For this review, use the dimensioned drawing (mm, ordinates from the lowest corner) and the shaded views. A direction names the side the tool comes from. Give positions to 0.01 mm unless a question says otherwise; leave off trailing zeros. Loops run counter-clockwise (first coordinate to the right, second up) from the corner with the lowest first, then second, coordinate; pieces in that order, holes last. Notation, with made-up numbers: M 76,59 L 119,59 A25 cw 119,86 Z; hole C 73.25,73.5 d6. An arc over 180 degrees is marked long. Return JSON: item names as keys, results as strings.
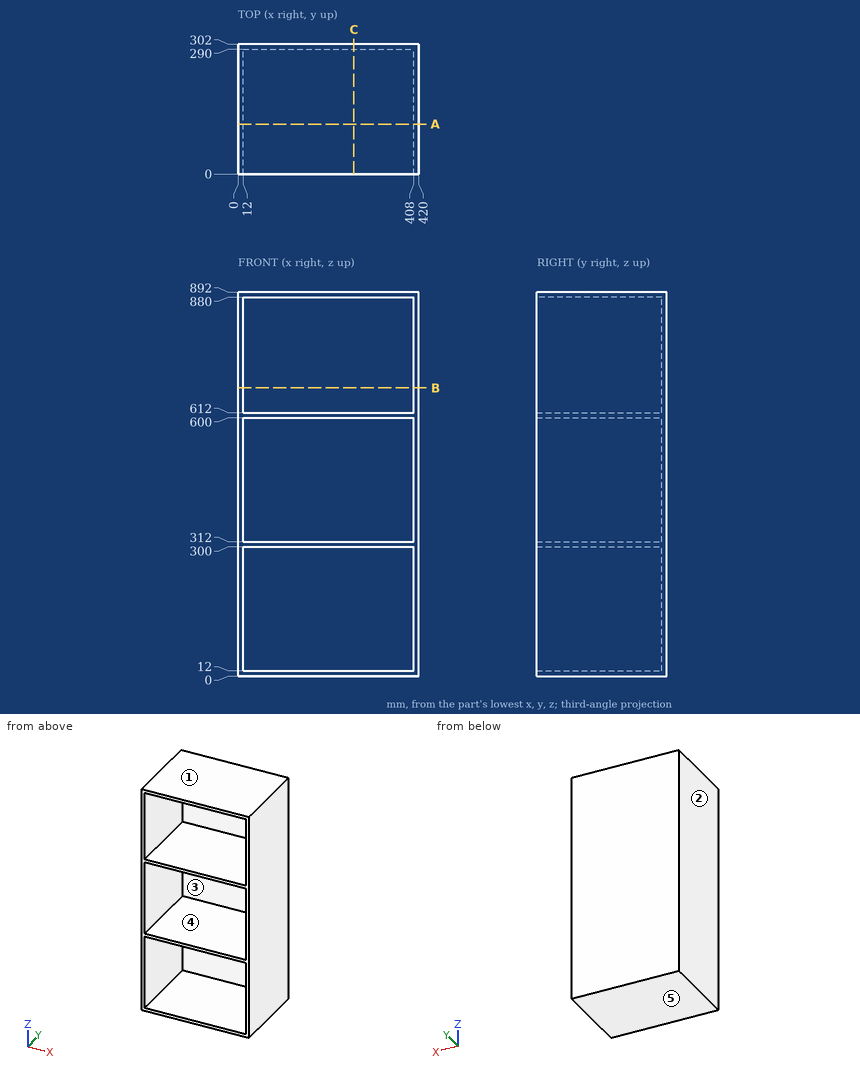
1) Consider section C-C on x = 269. Write out the cut boundary in (y, z).
From the geometry:
{"outline": "M 0,0 L 302,0 L 302,892 L 0,892 L 0,880 L 290,880 L 290,612 L 0,612 L 0,600 L 290,600 L 290,312 L 0,312 L 0,300 L 290,300 L 290,12 L 0,12 Z"}
2) Consider section B-B on z = 669.5. Write out the cut boundary in (x, y).
From the geometry:
{"outline": "M 0,0 L 12,0 L 12,290 L 408,290 L 408,0 L 420,0 L 420,302 L 0,302 Z"}
3) Tool access review of the marked faces 4 and 5: name each direction out of +Z, -Z, +X, -X, +Y, -Y from which nothing blocks a thin tool from reaching the whole face with its end or side.
From the geometry:
{"face 4": "-Y", "face 5": "-Z, +X, -X, +Y, -Y"}
4) Insertion check: pin 1 (1.5 mm diameter, centred on x = 259.5, y = 248, fed in from -Z); pin 2 (5 mm diameter, centred on x = 372.5, z = 712.5, fed in from -Y). Each pin has a flat end and moves straight along its axis. Give the tip position at first contact, or say it passes through.
From the geometry:
{"pin 1": "z = 0", "pin 2": "y = 290"}
5) Wall thickness on L1, parallel to Z at x = 64, y = 234; L2, parallel to X at y = 44.5, z = 856; L3, parallel to Y at x = 241, z = 378: over which ranges is each line inside the solid? List them lowest first. Write a range as from..to.
From the geometry:
{"L1": "0..12, 300..312, 600..612, 880..892", "L2": "0..12, 408..420", "L3": "290..302"}
6) The part is to be moulded in two halves that separate along Z. For the marked faces 1, 2 and 3, say which applies: released by +Z, released by -Z, zero draft, split by the parting line, or undercut.
From the geometry:
{"face 1": "released by +Z", "face 2": "zero draft", "face 3": "undercut"}
7) Consider section A-A on y = 116. Write out the cut boundary in (x, z).
From the geometry:
{"outline": "M 0,0 L 420,0 L 420,892 L 0,892 Z; hole M 12,12 L 408,12 L 408,300 L 12,300 Z; hole M 12,312 L 408,312 L 408,600 L 12,600 Z; hole M 12,612 L 408,612 L 408,880 L 12,880 Z"}
